Can you work these out from the drawing? Everything is in mm from the part's minimum corner. Round coordinates to 2 decimals unless told otherwise and drop trailing zeros. Loops run counter-clockwise (first coordinate to the right, second up) from the corner with the lowest first, then second, coordinate; pieces in that order, holes last. Notation, with made-up numbers: (13, 19) -> (48, 19) arc R26 ccw to (48, 46) -> close; hole circle Ø1 at (73.25, 41). An arc over 180 degrees is marked (long way). One line per item, written item: value.
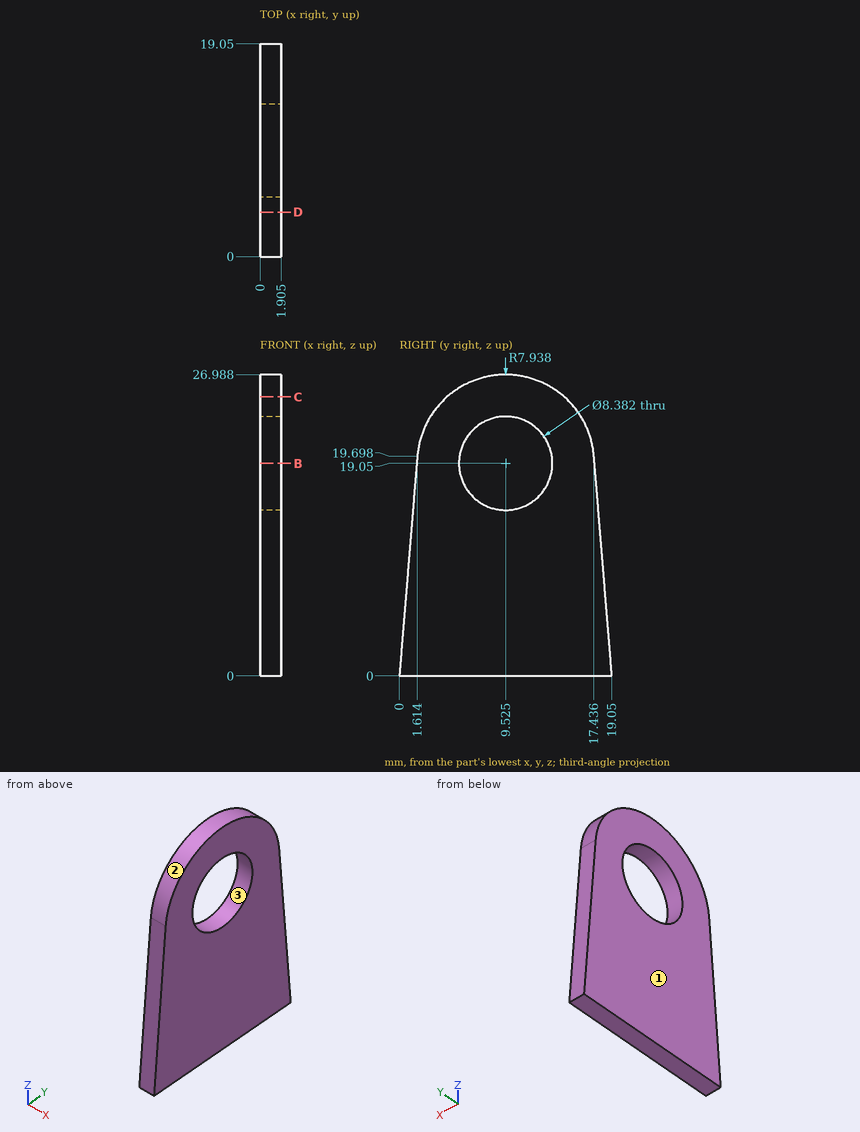
(1) If we section it at D-D, the plane y = 4: Please give me the cut outline in (x, z) (1 decimal).
Recorded:
outline: (0, 0) -> (1.9, 0) -> (1.9, 24.7) -> (0, 24.7) -> close
(2) Thinking about a two-plate mould opening in Y: for the marked faces 1, 2 and 3, which applies, released by +Y, released by -Y, zero draft, split by the parting line, or undercut?
Recorded:
face 1: zero draft
face 2: split by the parting line
face 3: undercut
(3) If I drill on L1, parallel to Z at x = 1.7, y = 8.25 (1 decimal); L2, parallel to Z at x = 1.65, y = 6 (1 decimal); L3, parallel to Z at x = 1, y = 15 (1 decimal), over which ranges is the centre line in solid material (lowest first)?
Recorded:
L1: 0 to 15.1, 23 to 26.9
L2: 0 to 16.8, 21.3 to 26.2
L3: 0 to 24.8
(4) I'm going to push a flat-ended pin straight in: pin 1 Ø1 at (x, z) = (1.5, 22.5) entering from -Y (1 decimal). Where does the tip first touch, or does it pass through?
Recorded:
pin 1: y = 2.2
(5) If we section it at B-B, the plane z = 19.05: Please give me the cut outline in (x, y) (1 decimal), then the cut area to 3 significant figures.
Recorded:
outline: (0, 1.6) -> (1.9, 1.6) -> (1.9, 5.3) -> (0, 5.3) -> close; (0, 13.7) -> (1.9, 13.7) -> (1.9, 17.5) -> (0, 17.5) -> close
area: 14.4 mm²
(6) If we section it at C-C, the plane z = 25: Please give me the cut outline in (x, y) (1 decimal).
Recorded:
outline: (0, 4.3) -> (1.9, 4.3) -> (1.9, 14.8) -> (0, 14.8) -> close
